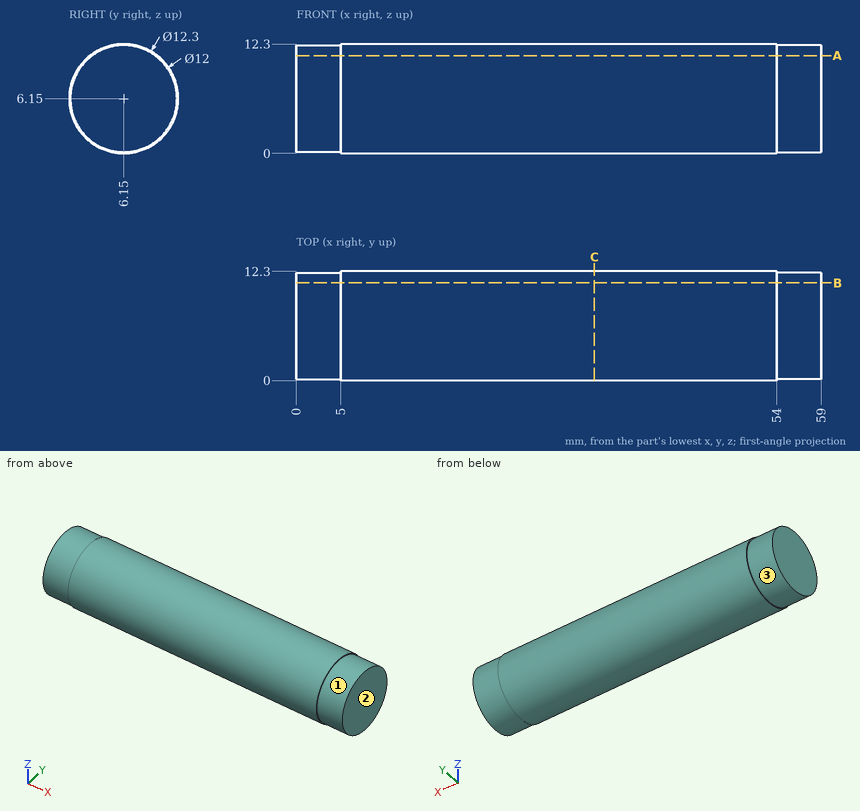
Geometry check sheet. Reference: drawing and pictorial views, mm from the part's lowest x, y, z. A direction names the side the tool comes from. Round coordinates to 2 decimals unless told otherwise and drop trailing zeros. Loops run counter-clockwise (first coordinate to the right, second up) from the corner with the lowest first, then second, coordinate; pieces in that order, holes last. Notation, with made-up numbers: M 55,15.5 L 102,15.5 A19 ccw 102,24.5 Z; hole C -4,59.5 d11. An arc over 180 degrees is marked long. Return JSON: item names as keys, results as strings. Group by question number.
(1) Section check A-A, the plane z = 11. Enter the section's corners in (x, y).
(2) Go/stop test with flat-tipped pins: pin 1 (3 mm diameter, centred on x = 28.5, z = 9, fed in from +Y); pin 2 (5 mm diameter, centred on y = 3.5, z = 3, fed in from -X); pin 3 (3 mm diameter, centred on x = 21.5, y = 11, fed in from -Z). Record where each tip stops, or that it passes through.
(3) Scan lines: line 1 along Z through (x, y) = (39, 6.5); line 2 along Y through (x, z) = (30, 4.75); line 3 along Z through (x, y) = (10.5, 3.75). Record each from-to range of solid material in increasing order. Write a range as [from, to].
(4) Set-up check for the marked faces 1, 2 and 3: record each of +Z, -Z, +X, -X, +Y, -Y from which the full face is reachable in a straight line by a thin tool's end or side.
(5) Section check C-C, the plane x = 33.5. Enter the section's corners in (y, z), and give its area (3 significant figures).
Data:
{
 "1": {"outline": "M 0,2.62 L 5,2.62 L 5,2.37 L 54,2.37 L 54,2.62 L 59,2.62 L 59,9.68 L 54,9.68 L 54,9.93 L 5,9.93 L 5,9.68 L 0,9.68 Z"},
 "2": {"pin 1": "y = 12.15", "pin 2": "x = 0", "pin 3": "z = 0.99"},
 "3": {"line 1": "[0.01, 12.29]", "line 2": "[0.16, 12.14]", "line 3": "[0.49, 11.81]"},
 "4": {"face 1": "+X", "face 2": "+Z, -Z, +X, +Y, -Y", "face 3": "-X"},
 "5": {"outline": "C 6.15,6.15 d12.3", "area": "119 mm²"}
}
